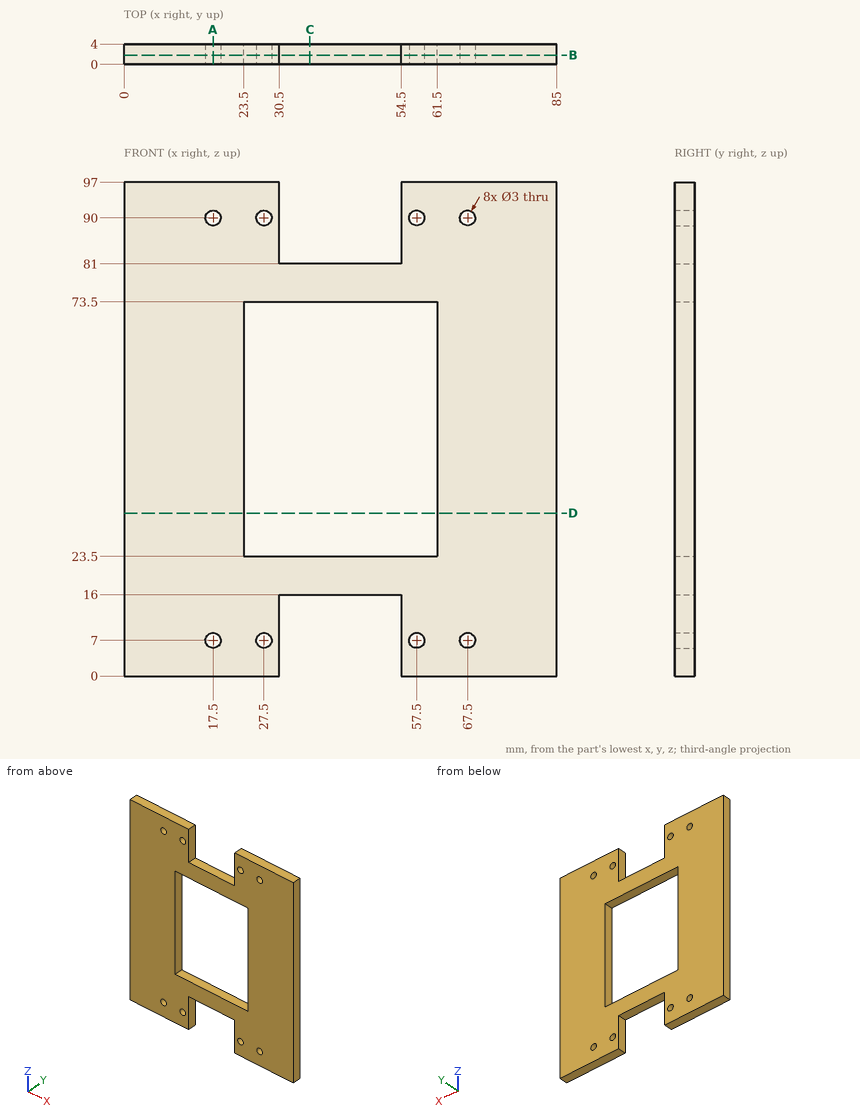
The drawing under review shows one solid part. Ordinate dimensions are in mm from its lowest x, y, z. Coordinates: 2 decimals unless noted, no trailing zeros. Write each loop counter-clockwise with the first axis right and the second up, starting at its lowest first coordinate (ties: lowest second). Pieces come first, ordered by that corner, then holes. Notation, with made-up numbers: (-19, -32) - (2, -32) arc R15 cw to (2, -7) - close; hole circle Ø11 at (15, 57). An arc over 180 degrees is marked (long way). Put each result on its own line as item: value.
1. Add section C-C, the plane x = 36.5. Give the boundary of the cut face in (y, z).
Values found:
outline: (0, 16) - (4, 16) - (4, 23.5) - (0, 23.5) - close; (0, 73.5) - (4, 73.5) - (4, 81) - (0, 81) - close
2. Wall thickness on probe 1 along X at (y, z) = (2.4, 7); probe 2 along X at (y, z) = (3.35, 54.5); probe 3 along Z at (x, y) = (60, 1.6): over which ranges is each line inside the solid? List them lowest first.
Values found:
probe 1: 0 to 16, 19 to 26, 29 to 30.5, 54.5 to 56, 59 to 66, 69 to 85
probe 2: 0 to 23.5, 61.5 to 85
probe 3: 0 to 23.5, 73.5 to 97
3. Add section A-A, the plane x = 17.5. Give the boundary of the cut face in (y, z).
Values found:
outline: (0, 0) - (4, 0) - (4, 5.5) - (0, 5.5) - close; (0, 8.5) - (4, 8.5) - (4, 88.5) - (0, 88.5) - close; (0, 91.5) - (4, 91.5) - (4, 97) - (0, 97) - close
4. Add section D-D, the plane z = 32. Give the boundary of the cut face in (x, y).
Values found:
outline: (0, 0) - (23.5, 0) - (23.5, 4) - (0, 4) - close; (61.5, 0) - (85, 0) - (85, 4) - (61.5, 4) - close
5. Add section B-B, the plane y = 1.8. Count the separate pieces of the cut face and the enclosed holes in it, then the cut area to 3 significant figures.
Values found:
separate pieces: 1
enclosed holes: 9
area: 5,520 mm²
6. For pin 1 (2.5 mm diameter, centred on x = 27.5, z = 7, fed in from +Y); pin 2 (2 mm diameter, centred on y = 2, z = 92.5, fed in from -X); pin 3 (2 mm diameter, centred on x = 46, y = 2.5, fed in from -Z), all flat-tipped, find the tip position at first contact; note any pin that passes through.
Values found:
pin 1: through
pin 2: x = 0
pin 3: z = 16
